from build123d import *

# Parameters (mm, degrees)
SKETCH1_W           = 9.5
SKETCH1_H           = 4.5
BOSS_EXTRUDE1_DEPTH = 5
SKETCH2_W           = 11
SKETCH2_H           = 6
BOSS_EXTRUDE2_DEPTH = 3
FILLET1_R           = 2
FILLET2_R           = 1


with BuildPart() as part:
    # Sketch1 → Boss-Extrude1 (new body)
    with BuildSketch(Plane.XY):
        with Locations((4.75, 2.25)):
            Rectangle(SKETCH1_W, SKETCH1_H)
    extrude(amount=BOSS_EXTRUDE1_DEPTH)

    # Sketch2 → Boss-Extrude2 (add)
    with BuildSketch(Plane.XY.offset(5)):
        with Locations((4.75, 2.25)):
            Rectangle(SKETCH2_W, SKETCH2_H)
    extrude(amount=BOSS_EXTRUDE2_DEPTH)

    # Fillet1
    fillet1_edges = [part.edges().sort_by_distance(p)[0] for p in [
        (0, 4.5, 2.5),
        (9.5, 4.5, 2.5),
        (9.5, 0, 2.5),
        (0, 0, 2.5),
    ]]
    fillet(fillet1_edges, radius=FILLET1_R)

    # Fillet2
    fillet2_edges = [part.edges().sort_by_distance(p)[0] for p in [
        (0, 2.25, 0),
        (4.75, 4.5, 0),
        (9.5, 2.25, 0),
        (4.75, 0, 0),
        (0.585786438, 0.585786438, 0),
        (8.914213562, 0.585786438, 0),
        (8.914213562, 3.914213562, 0),
        (0.585786438, 3.914213562, 0),
    ]]
    fillet(fillet2_edges, radius=FILLET2_R)


solid = part.part
Check sheet for the modelled part. Datum: model origin and axes. Units: mm. A direction names the side the tool comes from. Round coordinates to 2 decimals unless told otherwise and drop trailing zeros. Loops run counter-clockwise (first coordinate to the right, second up) from the corner with the lowest first, then second, coordinate; pieces in that order, holes last.
1. Sectioned sample at D-D on x = 9.75. Record the boundary of the cut face in (y, z), and give its area (3 significant figures).
2. Scan lines: probe 1 along X at (y, z) = (2.3, 1); probe 2 along Y at (x, z) = (2, 3.75); probe 3 along Z at (x, y) = (3.25, 4.7). Record each from-to range of solid material in increasing order.
3. Sectioned sample at A-A on x = 4. Record the boundary of the cut face in (y, z).
4. Sectioned sample at C-C on y = -0.2. Record the boundary of the cut face in (x, z), and give its area (3 significant figures).
5. Gauge pin test, flat ends, axial feed: pin 1 Ø1.2 at (x, z) = (3.5, 3.5) entering from +Y; pin 2 Ø1.5 at (x, y) = (2, 4.5) entering from -Z; pin 3 Ø4.5 at (x, z) = (3.5, 3) entering from -Y. Record the tip position at first contact, or that the pin passes through.
6. Sectioned sample at B-B on z = 2.75. Record the boundary of the cut face in (x, y), and give its area (3 significant figures).
7. Set-up check for faces 1 (the cylindrical face through (0.6, 3.93, 3.03)), 2 (the flat face through (5, 4.5, 3)), 3 (the flat face through (5, 5, 5)), 4 (the flat face through (5, 0, 3)): record each of +Z, -Z, +X, -X, +Y, -Y from which the full face is reachable in a straight line by a thin tool's end or side.
Recorded:
1. outline: (-0.75, 5) - (5.25, 5) - (5.25, 8) - (-0.75, 8) - close
1. area: 18.0 mm2
2. probe 1: x = 0 to 9.5
2. probe 2: y = 0 to 4.5
2. probe 3: z = 5 to 8
3. outline: (-0.75, 5) - (0, 5) - (0, 1) arc R1 ccw to (1, 0) - (3.5, 0) arc R1 ccw to (4.5, 1) - (4.5, 5) - (5.25, 5) - (5.25, 8) - (-0.75, 8) - close
4. outline: (-0.75, 5) - (10.25, 5) - (10.25, 8) - (-0.75, 8) - close
4. area: 33.0 mm2
5. pin 1: stops at y = 4.5
5. pin 2: stops at z = 0.03
5. pin 3: stops at y = -0.75
6. outline: (0, 2) arc R2 ccw to (2, 0) - (7.5, 0) arc R2 ccw to (9.5, 2) - (9.5, 2.5) arc R2 ccw to (7.5, 4.5) - (2, 4.5) arc R2 ccw to (0, 2.5) - close
6. area: 39.3 mm2
7. face 1: -Z, -X, +Y
7. face 2: -Z, +X, -X, +Y
7. face 3: -Z
7. face 4: -Z, +X, -X, -Y
